Check sheet for the modelled part. Datum: model origin and axes. Units: mm. Give positions to 0.01 mm unless a question says otherwise; leave off trailing zeros. Order: outer loops, then holes, each group sorted by start corner. A loop starts at its lowest first (then second) coordinate and runs counter-clockwise, first axis right, second up.
from build123d import *

# Parameters (mm, degrees)
SKETCH1_W           = 94
SKETCH1_H           = 123
SKETCH1_R           = 1.6
SKETCH1_W_2         = 4.6
SKETCH1_H_2         = 2.1
SKETCH1_W_3         = 2.1
SKETCH1_H_3         = 4.6
BOSS_EXTRUDE1_DEPTH = 1
FILLET1_R           = 1
CUT_EXTRUDE1_REACH  = 79.429
SKETCH2_R           = 5.05
SKETCH2_R_2         = 1.05
SKETCH2_W           = 3.2
SKETCH2_H           = 12


with BuildPart() as part:
    # Sketch1 → Boss-Extrude1 (new, symmetric)
    with BuildSketch(Plane.XY):
        Rectangle(SKETCH1_W, SKETCH1_H)
        with Locations((-44, 58.5)):
            Circle(SKETCH1_R, mode=Mode.SUBTRACT)
        with Locations(Location((-44, -58.5, 0), (0, 0, 180))):
            Circle(SKETCH1_R, mode=Mode.SUBTRACT)
        with Locations((44, -58.5)):
            Circle(SKETCH1_R, mode=Mode.SUBTRACT)
        with Locations(Location((44, 58.5, 0), (0, 0, 180))):
            Circle(SKETCH1_R, mode=Mode.SUBTRACT)
        with Locations((0, -58.45)):
            Rectangle(SKETCH1_W_2, SKETCH1_H_2, mode=Mode.SUBTRACT)
        with Locations((0, 58.45)):
            Rectangle(SKETCH1_W_2, SKETCH1_H_2, mode=Mode.SUBTRACT)
        with Locations((-43.95, -27.2)):
            Rectangle(SKETCH1_W_3, SKETCH1_H_3, mode=Mode.SUBTRACT)
        with Locations((-43.95, 27.2)):
            Rectangle(SKETCH1_W_3, SKETCH1_H_3, mode=Mode.SUBTRACT)
        with Locations((43.95, -27.2)):
            Rectangle(SKETCH1_W_3, SKETCH1_H_3, mode=Mode.SUBTRACT)
        with Locations((43.95, 27.2)):
            Rectangle(SKETCH1_W_3, SKETCH1_H_3, mode=Mode.SUBTRACT)
    extrude(amount=BOSS_EXTRUDE1_DEPTH, both=True)

    # Fillet1
    fillet1_edges = [part.edges().sort_by_distance(p)[0] for p in [
        (47, -61.5, 0),
        (-47, -61.5, 0),
        (-47, 61.5, 0),
        (47, 61.5, 0),
    ]]
    fillet(fillet1_edges, radius=FILLET1_R)

    # Sketch2 → Cut-Extrude1 (cut, up to next)
    with BuildSketch(Plane.XY.offset(1), mode=Mode.PRIVATE) as cut_extrude1_sk1:
        with Locations((27.890121282, -43.5)):
            Circle(SKETCH2_R)
    cut_extrude1_tool1 = extrude(cut_extrude1_sk1.sketch, amount=-CUT_EXTRUDE1_REACH, mode=Mode.PRIVATE) & part.part
    # Sketch2 → Cut-Extrude1 (cut, up to next)
    with BuildSketch(Plane.XY.offset(1), mode=Mode.PRIVATE) as cut_extrude1_sk2:
        with Locations((7.2, -23.2)):
            Circle(SKETCH2_R_2)
    cut_extrude1_tool2 = extrude(cut_extrude1_sk2.sketch, amount=-CUT_EXTRUDE1_REACH, mode=Mode.PRIVATE) & part.part
    # Sketch2 → Cut-Extrude1 (cut, up to next)
    with BuildSketch(Plane.XY.offset(1), mode=Mode.PRIVATE) as cut_extrude1_sk3:
        with Locations((31, -23.2)):
            Circle(SKETCH2_R_2)
    cut_extrude1_tool3 = extrude(cut_extrude1_sk3.sketch, amount=-CUT_EXTRUDE1_REACH, mode=Mode.PRIVATE) & part.part
    # Sketch2 → Cut-Extrude1 (cut, up to next)
    with BuildSketch(Plane.XY.offset(1), mode=Mode.PRIVATE) as cut_extrude1_sk4:
        with Locations((31, 0.1)):
            Circle(SKETCH2_R_2)
    cut_extrude1_tool4 = extrude(cut_extrude1_sk4.sketch, amount=-CUT_EXTRUDE1_REACH, mode=Mode.PRIVATE) & part.part
    # Sketch2 → Cut-Extrude1 (cut, up to next)
    with BuildSketch(Plane.XY.offset(1), mode=Mode.PRIVATE) as cut_extrude1_sk5:
        with Locations((7.2, 0.1)):
            Circle(SKETCH2_R_2)
    cut_extrude1_tool5 = extrude(cut_extrude1_sk5.sketch, amount=-CUT_EXTRUDE1_REACH, mode=Mode.PRIVATE) & part.part
    # Sketch2 → Cut-Extrude1 (cut, up to next)
    with BuildSketch(Plane.XY.offset(1), mode=Mode.PRIVATE) as cut_extrude1_sk6:
        with Locations((6.8, -11.55)):
            Rectangle(SKETCH2_W, SKETCH2_H)
    cut_extrude1_tool6 = extrude(cut_extrude1_sk6.sketch, amount=-CUT_EXTRUDE1_REACH, mode=Mode.PRIVATE) & part.part
    add(cut_extrude1_tool1.solids().sort_by_distance((27.890121, -43.5, 1))[0], mode=Mode.SUBTRACT)
    add(cut_extrude1_tool2.solids().sort_by_distance((7.2, -23.2, 1))[0], mode=Mode.SUBTRACT)
    add(cut_extrude1_tool3.solids().sort_by_distance((31, -23.2, 1))[0], mode=Mode.SUBTRACT)
    add(cut_extrude1_tool4.solids().sort_by_distance((31, 0.1, 1))[0], mode=Mode.SUBTRACT)
    add(cut_extrude1_tool5.solids().sort_by_distance((7.2, 0.1, 1))[0], mode=Mode.SUBTRACT)
    add(cut_extrude1_tool6.solids().sort_by_distance((6.8, -11.55, 1))[0], mode=Mode.SUBTRACT)


solid = part.part
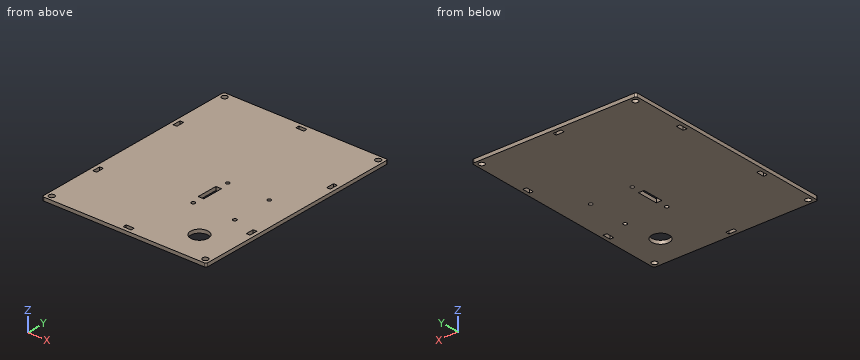
1) Section check D-D, the plane z = 0.65. State how many separate pieces and enclosed holes the cut face has, then the cut area to 3 significant figures.
Recorded:
separate pieces: 1
enclosed holes: 16
area: 11,300 mm2
2) Depth check by flat-ended pin: pin 1 Ø1.9 at (x, y) = (-44, 58.5) entering from -Z. Enter the tip coordinate at first touch or a pass-through.
Recorded:
pin 1: passes through
3) Section check B-B, the plane x = 27.5. Record the cut outline in (y, z), then the cut area to 3 significant figures.
Recorded:
outline: (-61.5, -1) - (-48.53, -1) - (-48.53, 1) - (-61.5, 1) - close; (-38.47, -1) - (61.5, -1) - (61.5, 1) - (-38.47, 1) - close
area: 226 mm2
4) Section check A-A, the plane y = -27.5. Record the cut outline in (x, z).
Recorded:
outline: (-47, -1) - (-45, -1) - (-45, 1) - (-47, 1) - close; (-42.9, -1) - (42.9, -1) - (42.9, 1) - (-42.9, 1) - close; (45, -1) - (47, -1) - (47, 1) - (45, 1) - close
5) Section check C-C, the plane y = -8. Record the cut outline in (x, z).
Recorded:
outline: (-47, -1) - (5.2, -1) - (5.2, 1) - (-47, 1) - close; (8.4, -1) - (47, -1) - (47, 1) - (8.4, 1) - close
6) Material ranges on L1, parallel to Y at x = 7.2, z = -0.1; L2, parallel to Y at x = -44, z = -0.2; L3, parallel to X at y = -6.5, z = 0.7, recorded low to high.
Recorded:
L1: y = -61.5 to -24.25, -22.15 to -17.55, -5.55 to -0.95, 1.15 to 61.5
L2: y = -61.5 to -60.1, -56.9 to -29.5, -24.9 to 24.9, 29.5 to 56.9, 60.1 to 61.5
L3: x = -47 to 5.2, 8.4 to 47
